Read the model definition and answer for the solid it produces. Units are mm, in the model's axes. A direction names the side the tool comes from. Round coordinates to 2 decimals unless told otherwise and drop trailing zeros. Order: outer loops, then holes, each group sorted by start corner. A loop starts at its lowest first (then second) coordinate and runs counter-clockwise, first axis right, second up. Notation, with made-up numbers: (46.5, -36.75) -> (98.5, -36.75) arc R28 ccw to (98.5, -5.75) -> close; hole circle Ø11 at (9.5, -24). An arc over 180 degrees is marked (long way). Answer as a JSON object with one key per item and string values. Group by question number.
Item 1: Section A-A, the plane y = 0 is taken. Write down the section's boundary in (x, z) (3 decimals), plus the area to 3 significant figures.
Item 2: Given P1, Ø1, axis at x = 7.5, z = 14, coming from the -Y side; P2, Ø4, axis at x = 2.5, z = 15, coming from the -Y side; P3, Ø8, axis at x = -6.5, y = -4.5, coming from the -Z side; P4, Ø4.5, axis at y = 0, z = 9.525, coming from the -X side, each flat-ended and moving along its own axis, determine where each tip first touches the part or whether it passes through.
Item 3: Consider probe 1 along Z at (x, y) = (5.75, 0); probe 2 along Z at (x, y) = (-5.25, -5); probe 3 along Y at (x, z) = (0, 17) (3 decimals). Determine where each line is inside the solid, lowest interval first. Write a range as from..to.
Item 4: Section B-B, the plane z = 15 is taken. Write down the section's boundary in (x, y) (3 decimals), plus the area to 3 significant figures.
Item 5: For faces 1 (the cylindrical face through (-0.69, -3.1, 20.49)), 2 (the cylindrical face through (8.8, -3.65, 9.4)), 3 (the cylindrical face through (-0.69, -3.1, -1.44)), determine the directions among +Z, -Z, +X, -X, +Y, -Y from which every point of the face is accessible in a straight line to the end or side of a thin tool.
from build123d import *

# Parameters (mm, degrees)
F0_R     = 9.525
F1_DEPTH = 19.05
F2_R     = 3.175
F3_DEPTH = 3.175
F4_R     = 3.175
F5_DEPTH = 3.175
F6_SIZE  = 0.254
F7_R     = 2.794
F8_DEPTH = 25.4
F9_DEPTH = 25.4


with BuildPart() as f1:
    # F0 (on Top) → F1 (new body)
    with BuildSketch(Plane.XY):
        Circle(F0_R)
    extrude(amount=F1_DEPTH)

    # F2 (on Top) → F3 (join)
    with BuildSketch(Plane.XY):
        Circle(F2_R)
    extrude(amount=-F3_DEPTH)

    # F4 (on face) → F5 (join)
    with BuildSketch(Plane.XY.offset(19.05)):
        Circle(F4_R)
    extrude(amount=F5_DEPTH)

    # F6
    f6_edges = [f1.edges().sort_by_distance(p)[0] for p in [
        (-3.175, 0, 22.225),
        (-9.525, 0, 19.05),
        (-3.175, 0, -3.175),
        (-9.525, 0, 0),
    ]]
    chamfer(f6_edges, length=F6_SIZE)

    # F7 (on Right) → F8 (cut)
    with BuildSketch(Plane.YZ):
        with Locations((0, 9.525)):
            Circle(F7_R)
    extrude(amount=-F8_DEPTH, mode=Mode.SUBTRACT)

    # F7 (on Right) → F9 (cut)
    with BuildSketch(Plane.YZ):
        with Locations((0, 9.525)):
            Circle(F7_R)
    extrude(amount=F9_DEPTH, mode=Mode.SUBTRACT)


solid = f1.part
Values found:
{
 "1": {"outline": "(-9.525, 0.254) -> (-9.271, 0) -> (-3.175, 0) -> (-3.175, -2.921) -> (-2.921, -3.175) -> (2.921, -3.175) -> (3.175, -2.921) -> (3.175, 0) -> (9.271, 0) -> (9.525, 0.254) -> (9.525, 6.731) -> (-9.525, 6.731) -> close; (-9.525, 12.319) -> (9.525, 12.319) -> (9.525, 18.796) -> (9.271, 19.05) -> (3.175, 19.05) -> (3.175, 21.971) -> (2.921, 22.225) -> (-2.921, 22.225) -> (-3.175, 21.971) -> (-3.175, 19.05) -> (-9.271, 19.05) -> (-9.525, 18.796) -> close", "area": "297 mm2"},
 "2": {"P1": "y = -6.46", "P2": "y = -9.51", "P3": "z = 0", "P4": "through"},
 "3": {"probe 1": "0..6.73, 12.32..19.05", "probe 2": "0..19.05", "probe 3": "-9.525..9.525"},
 "4": {"outline": "circle Ø19.05 at (0, 0)", "area": "285 mm2"},
 "5": {"face 1": "+Z", "face 2": "+Z, -Z", "face 3": "-Z"}
}
